Input: part model. Units: mm. Frame: model coordinates. Face numbers are marked on the shaded views. A direction names the side the tool comes from. Round coordinates to 2 decimals unless told otherwise and drop trailing zeros. Loops run counter-clockwise (first coordinate to the right, second up) from the corner with the lowest first, then second, coordinate; pieces in that order, holes last. Notation, with made-up numbers: (42, 50) -> (97, 50) arc R22 cw to (97, 67) -> close; hole circle Ø7 at (3, 80). An arc over 180 degrees is marked (long way). Answer as a JSON object with one key per item and string values. Group by question number.
Item 1: Set-up query: the marked faces 1, 2, 3, 4 and 5. Return all of +Z, -Z, +X, -X, +Y, -Y with unobstructed straight access to the full face (end or side cutting, diameter ignored); none if empty.
Item 2: Section query D-D on x = -13.5. Return loops of the section in (y, z).
Item 3: Material intervals for line 1 (X direction, y = 19, z = -3.5); line 2 (X direction, y = -4.5, z = 12); line 3 (Z direction, x = -31, y = 6.5), sorted ascending. Write a range as [from, to].
Item 4: Pin query (flat end, axial travel): pin 1 (4 mm diameter, centred on x = -18.5, z = 8.5, fed in from +Y); pin 2 (1.2 mm diameter, centred on x = -18.5, z = -2.5, fed in from +Y); pin 3 (5.5 mm diameter, centred on y = -5, z = 2, fed in from +X). Return the tip coordinate at first contact, or that it passes through.
Item 5: Section query B-B on z = 12.5. Return loops of the section in (x, y), and give its area (3 significant figures).
Item 6: Draft query along Z for the marked faces 6, 7 and 8. Return one class per face: released by +Z, released by -Z, zero draft, split by the parting line, or undercut.
Item 7: Section query C-C on y = 11. Return loops of the section in (x, z), and give its area (3 significant figures).
Item 8: Section query A-A on y = 29. Return loops of the section in (x, z).
Autodesk Inventor part; units mm, degrees
ref_plane "YZ Plane" through (0, 0, 0) normal (1, 0, 0) x (0, 1, 0)
ref_plane "XZ Plane" through (0, 0, 0) normal (0, 1, 0) x (-1, 0, 0)
ref_plane "XY Plane" through (0, 0, 0) normal (0, 0, 1) x (1, 0, 0)
sketch "스케치1" plane through (0, 0, 0) normal (0, 1, 0) x (-1, 0, 0)
  line L0 (0, 0) -> (32.6, 0)
  line L1 (32.6, 0) -> (32.6, -2)
  line L2 (0, -2) -> (0, 0)
  line L3 (34.6, -4) -> (34.6, 2)
  line L4 (34.6, 2) -> (-2, 2)
  line L5 (-2, 2) -> (-2, -4)
  line L6 (26.6, -2) -> (26.6, -4)
  line L7 (6, -2) -> (6, -4)
  line L8 (32.6, -2) -> (26.6, -2)
  line L9 (6, -2) -> (0, -2)
  line L10 (-2, -4) -> (6, -4)
  line L11 (26.6, -4) -> (34.6, -4)
  dimension "d0" = 32.6
  dimension "d1" = 2
  dimension "d3" = 6
  dimension "d4" = 6
extrude "돌출1" add sketch "스케치1" along normal blind 32.6
sketch "스케치2" plane through (0, 0, 0) normal (0, -1, 0) x (1, 0, 0)
  line L0 (0, -2) -> (0, 0)
  line L1 (-6, -2) -> (0, -2)
  line L2 (-6, -4) -> (-6, -2)
  line L3 (2, -4) -> (-6, -4)
  line L4 (2, 2) -> (2, -4)
  line L5 (-34.6, 2) -> (2, 2)
  line L6 (-34.6, -4) -> (-34.6, 2)
  line L7 (-26.6, -4) -> (-34.6, -4)
  line L8 (-26.6, -2) -> (-26.6, -4)
  line L9 (-32.6, -2) -> (-26.6, -2)
  line L10 (-32.6, 0) -> (-32.6, -2)
  line L11 (0, 0) -> (-32.6, 0)
  line L12 (-6, -4) -> (-6, -2)
  line L13 (-6, -4) -> (-26.6, -4)
extrude "돌출2" add sketch "스케치2" along normal blind 2
sketch "스케치3" plane through (-34.6, 32.6, 2) normal (0, 0, 1) x (1, 0, 0)
  line L0 (2, -32.6) -> (2, 0)
  line L1 (2, 0) -> (10, 0)
  line L2 (10, 0) -> (10, -25)
  line L3 (10, -25) -> (2, -25)
  line L4 (2, -25) -> (2, 0)
  line L5 (0, 0) -> (36.6, 0)
  point P0 (34.6, -32.6)
  point P1 (2, -25)
  dimension "d9" = 8
  dimension "d10" = 25
extrude "돌출3" cut sketch "스케치3" against normal blind 2
sketch "스케치4" plane through (0, -2, 0) normal (0, -1, 0) x (1, 0, 0)
  line L0 (-9.3, 15) -> (-23.3, 15)
  line L1 (-23.3, 15) -> (-23.3, -15)
  line L2 (-23.3, -15) -> (-9.3, -15)
  line L3 (-9.3, -15) -> (-9.3, 15)
  line L4 (-34.6, -4) -> (2, -4)
  line L5 (-9.3, 15) -> (-11.3, 15)
  line L6 (-11.3, 15) -> (-11.3, -15)
  line L7 (-11.3, -15) -> (-9.3, -15)
  line L8 (-9.3, -15) -> (-9.3, 15)
  line L9 (-23.3, -15) -> (-21.3, -15)
  line L10 (-21.3, -15) -> (-21.3, 15)
  line L11 (-21.3, 15) -> (-23.3, 15)
  line L12 (-23.3, 15) -> (-23.3, -15)
  line L13 (-21.3, 15) -> (-23.3, 15)
  line L14 (-23.3, 15) -> (-23.3, -15)
  line L15 (-23.3, -15) -> (-21.3, -15)
  line L16 (-21.3, -15) -> (-21.3, 15)
  point P0 (0, 0)
  point P1 (-16.3, -15)
  point P2 (-16.3, -4)
  point P3 (-9.3, 0)
  point P4 (-21.3, -4)
  point P5 (-23.3, -4)
  point P6 (-21.3, -4)
  dimension "d13" = 14
  dimension "d14" = 30
  dimension "d15" = 2
  dimension "d16" = 2
extrude "돌출4" add sketch "스케치4" along normal blind 2
extrude "돌출5" add sketch "스케치4" along normal blind 5 contours L3 L4 L6 L0 | L3 L2 L6 L4 | L10 L4 L1 L0
extrude "돌출6" add sketch "스케치4" along normal blind 5 contours L10 L2 L1 L4
sketch "스케치5" plane through (-34.6, 32.6, 2) normal (0, 0, 1) x (1, 0, 0)
  line L0 (28.6, 0) -> (34.6, 0)
  line L1 (34.6, 0) -> (29.6, 0)
  line L2 (29.6, 0) -> (29.6, -20)
  line L3 (29.6, -20) -> (34.6, -20)
  line L4 (34.6, -20) -> (34.6, 0)
  point P0 (34.6, -32.6)
  dimension "d23" = 5
  dimension "d24" = 20
extrude "돌출7" cut sketch "스케치5" against normal blind 2
fillet "모깎기1" radius 2 2 edges at (-5, 32.6, 1) (-24.6, 32.6, 1)
properties part number "end effector"
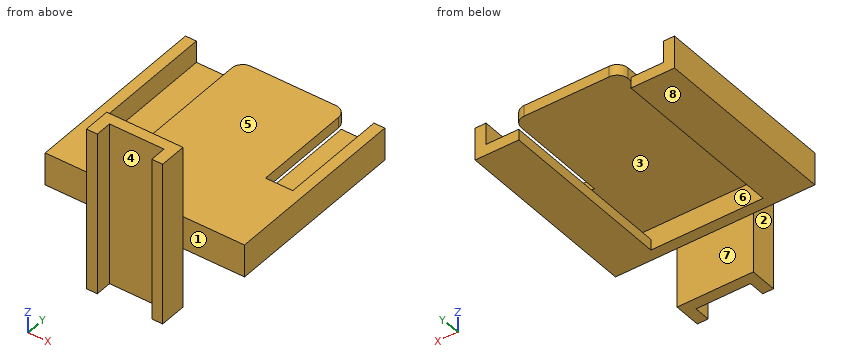
Solved:
{
 "1": {"face 1": "+Z, -Z, +X, -Y", "face 2": "+Z, -Z, -X, -Y", "face 3": "+Y", "face 4": "+Z, -Z, -Y", "face 5": "+Z, +X, -X, +Y"},
 "2": {"outline": "(-4, -15) -> (-2, -15) -> (-2, -4) -> (0, -4) -> (0, 0) -> (32.6, 0) -> (32.6, 2) -> (-2, 2) -> (-2, 15) -> (-4, 15) -> close"},
 "3": {"line 1": "[-34.6, -26.6], [-6, 2]", "line 2": "[-23.3, -21.3], [-11.3, -9.3]", "line 3": "[-4, -2], [0, 2]"},
 "4": {"pin 1": "y = -2", "pin 2": "y = 0", "pin 3": "x = -9.3"},
 "5": {"outline": "(-23.3, -7) -> (-21.3, -7) -> (-21.3, -4) -> (-11.3, -4) -> (-11.3, -7) -> (-9.3, -7) -> (-9.3, -2) -> (-23.3, -2) -> close", "area": "40.0 mm²"},
 "6": {"face 6": "undercut", "face 7": "zero draft", "face 8": "released by -Z"},
 "7": {"outline": "(-34.6, -4) -> (-26.6, -4) -> (-26.6, -2) -> (-32.6, -2) -> (-32.6, 2) -> (-34.6, 2) -> close; (-24.6, 0) -> (0, 0) -> (0, -2) -> (-6, -2) -> (-6, -4) -> (2, -4) -> (2, 2) -> (-24.6, 2) -> close", "area": "97.2 mm²"},
 "8": {"outline": "(-34.6, -4) -> (-26.6, -4) -> (-26.6, -2) -> (-32.6, -2) -> (-32.6, 2) -> (-34.6, 2) -> close; (-24.6, 0) -> (-5, 0) -> (-5, 2) -> (-24.6, 2) -> close; (-6, -4) -> (2, -4) -> (2, 2) -> (0, 2) -> (0, -2) -> (-6, -2) -> close"}
}
